from build123d import *

# Parameters (mm, degrees)
EXTRUDE_1_DEPTH     = 191
SKETCH_2_R          = 4.25
CUT_EXTRUDE_1_DEPTH = 21
SKETCH_3_R          = 2.25
CUT_EXTRUDE_2_DEPTH = 3


with BuildPart() as part:
    # Эскиз1 → Бобышка-Вытянуть1 (new body)
    with BuildSketch(Plane(origin=(0, 0, 0), x_dir=(1, 0, 0), z_dir=(0, 1, 0))):
        Polygon((0, 0), (0, 20), (2, 20), (2, 2), (40, 2), (40, 0), align=None)
    extrude(amount=EXTRUDE_1_DEPTH)

    # Эскиз2 → Вырез-Вытянуть1 (cut, through all)
    with BuildSketch(Plane.XY):
        with Locations((20, 130.5)):
            Circle(SKETCH_2_R)
        with Locations((20, 60.5)):
            Circle(SKETCH_2_R)
    extrude(amount=-CUT_EXTRUDE_1_DEPTH, mode=Mode.SUBTRACT)

    # Эскиз3 → Вырез-Вытянуть2 (cut, through all)
    with BuildSketch(Plane(origin=(2, 0, 0), x_dir=(0, 0, -1), z_dir=(1, 0, 0))):
        with Locations((10, 12)):
            Circle(SKETCH_3_R)
        with Locations((10, 179)):
            Circle(SKETCH_3_R)
    extrude(amount=-CUT_EXTRUDE_2_DEPTH, mode=Mode.SUBTRACT)


solid = part.part
The model under review builds one solid part; all positions refer to its coordinate system, in mm. A direction names the side the tool comes from. Round coordinates to 2 decimals unless told otherwise and drop trailing zeros. Order: outer loops, then holes, each group sorted by start corner. A loop starts at its lowest first (then second) coordinate and runs counter-clockwise, first axis right, second up. Notation, with made-up numbers: (19.5, 44) -> (75.5, 44) arc R12 cw to (75.5, 50) -> close; hole circle Ø9 at (-1.5, 34). An arc over 180 degrees is marked (long way). Use CSV: the item, a comma, the result in double quotes. Start each with the question number.
(1) Insertion check: pin 1 (12 mm diameter, centred on y = 81, z = -4.5, fed in from +X); pin 2 (11 mm diameter, centred on x = 20, y = 130.5, fed in from -Z); pin 3 (9 mm diameter, centred on y = 117.5, z = -12.5, fed in from +X). Each pin has a flat end and moves straight along its axis. Give the tip position at first contact, or say it passes through.
(2) Consider section B-B on x = 20. Write out the cut boundary in (y, z), and give its area (3 significant figures).
(3) Tool access review of faces 4 (the face through (20, 94, 0)), 5 (the face through (2, 94, -11)): name each direction out of +Z, -Z, +X, -X, +Y, -Y from which nothing blocks a thin tool from reaching the whole face with its end or side.
(4) Consider section A-A on y = 179. Write out the cut boundary in (x, z), and give its area (3 significant figures).
(5) Wall thickness on probe 1 along Y at (x, z) = (1.5, -10); probe 2 along Y at (x, z) = (20, -1.4); probe 3 along Z at (x, y) = (1.65, 179): over which ranges is each line inside the solid? List them lowest first. Write a range as from..to.
(6) Consider section D-D on y = 120. Write out the cut boundary in (x, z).
(7) Consider section C-C on z = -9.5. Write out the cut boundary in (x, y), and give its area (3 significant figures).
(8) Mouldability with a two-part tool opening along X and no side actions: class faces 1 (the face through (16, 191, -1)), 2 (the face through (19.447, 134.714, -0.986)), 3 (the face through (0, 94, -10)) as pulls with the +X half, pulls with the -X half, needs draft (parallel to the pull), parting line crosses it, or undercut.
Responses:
1,pin 1,"x = 40"
1,pin 2,"z = -2"
1,pin 3,"x = 2"
2,outline,"(0, -2) -> (56.25, -2) -> (56.25, 0) -> (0, 0) -> close; (64.75, -2) -> (126.25, -2) -> (126.25, 0) -> (64.75, 0) -> close; (134.75, -2) -> (191, -2) -> (191, 0) -> (134.75, 0) -> close"
2,area,"348 mm²"
3,face 4,"+Z, +X, -X, +Y, -Y"
3,face 5,"-Z, +X, +Y, -Y"
4,outline,"(0, -20) -> (2, -20) -> (2, -12.25) -> (0, -12.25) -> close; (0, -7.75) -> (2, -7.75) -> (2, -2) -> (40, -2) -> (40, 0) -> (0, 0) -> close"
4,area,"107 mm²"
5,probe 1,"0..9.75, 14.25..176.75, 181.25..191"
5,probe 2,"0..56.25, 64.75..126.25, 134.75..191"
5,probe 3,"-20..-12.25, -7.75..0"
6,outline,"(0, -20) -> (2, -20) -> (2, -2) -> (40, -2) -> (40, 0) -> (0, 0) -> close"
7,outline,"(0, 0) -> (2, 0) -> (2, 9.81) -> (0, 9.81) -> close; (0, 14.19) -> (2, 14.19) -> (2, 176.81) -> (0, 176.81) -> close; (0, 181.19) -> (2, 181.19) -> (2, 191) -> (0, 191) -> close"
7,area,"364 mm²"
8,face 1,"needs draft"
8,face 2,"undercut"
8,face 3,"pulls with the -X half"
